Model file for the job. Use its own axes, mm. A direction names the side the tool comes from. Round coordinates to 2 decimals unless told otherwise and drop trailing zeros. Order: outer loops, then holes, each group sorted by start corner. A loop starts at its lowest first (then second) coordinate and runs counter-clockwise, first axis right, second up. Notation, with made-up numbers: (20.25, 33) - (63.25, 33) arc R12 cw to (63.25, 48) - close; hole circle Ø7 at (-4.5, -27). An arc over 180 degrees is marked (long way). Write item = value, one per line. Start each with the question number.
from build123d import *

# Parameters (mm, degrees)
BOSS_EXTRUDE1_DEPTH     = 618.75
CUT_EXTRUDE1_DEPTH      = 10
BOSS_EXTRUDE5_DEPTH     = 2.5
CUT_EXTRUDE2_DEPTH      = 663.834510593
CUT_EXTRUDE2_DEPTH_BACK = 663.834510593
SKETCH5_R               = 6


with BuildPart() as part:
    # Sketch1 → Boss-Extrude1 (new, symmetric)
    with BuildSketch(Plane.XY):
        Polygon((-17.90633676, 20.183505355), (-17.90633676, -22.316494645), (-15.40633676, -22.316494645), (-15.40633676, 17.683505355), (24.59366324, 17.683505355), (24.59366324, 20.183505355), align=None)
    extrude(amount=BOSS_EXTRUDE1_DEPTH, both=True)

    # Sketch2 → Cut-Extrude1 (cut)
    with BuildSketch(Plane(origin=(0, 20.183505355, 0), x_dir=(1, 0, 0), z_dir=(0, 1, 0))):
        Polygon((-17.90633676, 618.75), (24.59366324, 576.25), (24.59366324, 618.75), align=None)
        Polygon((24.59366324, -576.25), (24.59366324, -618.75), (-17.90633676, -618.75), align=None)
    extrude(amount=-CUT_EXTRUDE1_DEPTH, mode=Mode.SUBTRACT)

    # Sketch3 → Boss-Extrude5 (add)
    with BuildSketch(Plane(origin=(-15.40633676, 0, 0), x_dir=(0, 0, -1), z_dir=(1, 0, 0))):
        Polygon((-616.25, 20.183505355), (-661.25, -22.316494645), (-616.25, -22.316494645), align=None)
        Polygon((616.25, 20.183505355), (661.25, -22.316494645), (616.25, -22.316494645), align=None)
    extrude(amount=-BOSS_EXTRUDE5_DEPTH)

    # Sketch5 → Cut-Extrude2 (cut, two sides: drawn at the far end of the back side and taken through both)
    with BuildSketch(Plane(origin=(-15.40633676, 0, 0), x_dir=(0, 0, -1), z_dir=(1, 0, 0)).offset(-CUT_EXTRUDE2_DEPTH_BACK)):
        with Locations(Location((-590, -7.316494645, 0), (0, 0, 90))):
            Circle(SKETCH5_R)
        with Locations(Location((-472, -7.316494645, 0), (0, 0, 90))):
            Circle(SKETCH5_R)
        with Locations(Location((-354, -7.316494645, 0), (0, 0, 90))):
            Circle(SKETCH5_R)
        with Locations(Location((-236, -7.316494645, 0), (0, 0, 90))):
            Circle(SKETCH5_R)
        with Locations(Location((-118, -7.316494645, 0), (0, 0, 90))):
            Circle(SKETCH5_R)
        with Locations(Location((0, -7.316494645, 0), (0, 0, 90))):
            Circle(SKETCH5_R)
        with Locations(Location((118, -7.316494645, 0), (0, 0, 90))):
            Circle(SKETCH5_R)
        with Locations(Location((236, -7.316494645, 0), (0, 0, 90))):
            Circle(SKETCH5_R)
        with Locations(Location((354, -7.316494645, 0), (0, 0, 90))):
            Circle(SKETCH5_R)
        with Locations(Location((472, -7.316494645, 0), (0, 0, 90))):
            Circle(SKETCH5_R)
        with Locations(Location((590, -7.316494645, 0), (0, 0, 90))):
            Circle(SKETCH5_R)
    extrude(amount=CUT_EXTRUDE2_DEPTH + CUT_EXTRUDE2_DEPTH_BACK, mode=Mode.SUBTRACT)


solid = part.part
Item 1: Saw through at B-B, the plane x = 14. Give the cut face in (y, z).
Item 2: Which spindle directions (+Z, -Z, +X, -X, +Y, -Y) get a long thin tool onto all of the face, cutting with end or side? Do faces 1 (the face through (4, 20.184, 9)), 2 (the face through (4, 17.684, 9)). Say none if no direction does.
Item 3: Probe L1, parallel to Y at x = -17.05, z = -590; L2, parallel to X at y = -14.5, z = -59; L3, parallel to Y at x = 3, z = -516.5. List the from-to ranges inside material, lowest first.
Item 4: Drop flat-ended pins along their axis: pin 1 (1.5 mm diameter, centred on y = -9, z = 173.5, fed in from +X); pin 2 (4 mm diameter, centred on x = -7, z = 363, fed in from -Y). Give the stop position or say it passes through.
Item 5: Saw through at A-A, the plane z = 518. Give the cut face in (x, y), then the cut area to 3 significant figures.
Check sheet entries:
q1.outline = (17.68, -586.84) - (20.18, -586.84) - (20.18, 586.84) - (17.68, 586.84) - close
q2.face_1 = +Z, -Z, +X, -X, +Y
q2.face_2 = +Z, -Z, +X, -Y
q3.L1 = -22.32 to -13.32, -1.32 to 20.18
q3.L2 = -17.91 to -15.41
q3.L3 = 17.68 to 20.18
q4.pin_1 = -15.41
q4.pin_2 = 17.68
q5.outline = (-17.91, -22.32) - (-15.41, -22.32) - (-15.41, 17.68) - (24.59, 17.68) - (24.59, 20.18) - (-17.91, 20.18) - close
q5.area = 206 mm2
